Autodesk Inventor part; units mm, degrees
ref_plane "YZ Plane" through (0, 0, 0) normal (1, 0, 0) x (0, 1, 0)
ref_plane "XZ Plane" through (0, 0, 0) normal (0, 1, 0) x (-1, 0, 0)
ref_plane "XY Plane" through (0, 0, 0) normal (0, 0, 1) x (1, 0, 0)
sketch "Sketch1" plane through (0, 0, 0) normal (0, 0, 1) x (1, 0, 0)
  line L0 (-300, 620) -> (300, 620)
  line L1 (300, 620) -> (300, 0)
  line L2 (300, 0) -> (-300, 0)
  line L3 (-300, 0) -> (-300, 620)
  point P0 (0, 0)
  point P1 (0, 0)
  dimension "d0" = 600
  dimension "d1" = 620
extrude "Extrusion1" add sketch "Sketch1" along normal blind 400
sketch "Sketch2" plane through (0, 0, 400) normal (0, 0, 1) x (1, 0, 0)
  line L0 (-300, 0) -> (300, 0)
  line L1 (300, 0) -> (300, 620)
  line L2 (300, 620) -> (-300, 620)
  line L3 (-300, 620) -> (-300, 0)
  line L4 (-275, 595) -> (275, 595)
  line L5 (275, 595) -> (275, 421.6667)
  line L6 (275, 421.6667) -> (-275, 421.6667)
  line L7 (-275, 421.6667) -> (-275, 595)
  line L8 (275, 396.6667) -> (-275, 396.6667)
  line L9 (-275, 396.6667) -> (-275, 223.3333)
  line L10 (-275, 223.3333) -> (275, 223.3333)
  line L11 (275, 223.3333) -> (275, 396.6667)
  line L12 (-275, 198.3333) -> (275, 198.3333)
  line L13 (275, 198.3333) -> (275, 25)
  line L14 (275, 25) -> (-275, 25)
  line L15 (-275, 25) -> (-275, 198.3333)
  line L16 (-275, 421.6667) -> (-275, 396.6667) construction
  line L17 (-275, 223.3333) -> (-275, 198.3333) construction
  line L18 (-275, 595) -> (-300, 620) construction
  line L19 (275, 595) -> (300, 620) construction
  line L20 (-275, 25) -> (-300, 0) construction
  point P0 (0, 0)
  dimension "d4" = 25
  dimension "d5" = 25
extrude "Extrusion2" cut sketch "Sketch2" against normal blind 375 contours L4 L5 L6 L7 | L11 L10 L9 L8 | L12 L13 L14 L15
equation "\"d5\" = d4"
equation "\"d6\" = d2 - d4"
properties part number "Pensile"
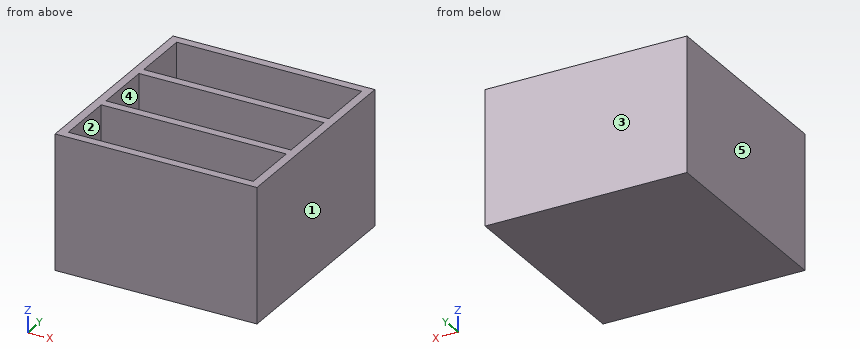
Geometry check sheet. Reference: the model listing, model coordinates, mm. Face numbers are marked on the shaded views. A direction names the side the tool comes from. Round coordinates to 2 decimals unless told otherwise and drop trailing zeros. Order: outer loops, then holes, each group sorted by start corner. A loop starts at its lowest first (then second) coordinate and runs counter-clockwise, first axis right, second up. Notation, with made-up numbers: M -19,-36 L 8,-36 A23 cw 8,-15 Z; hole C 35.25,13.25 d3. An arc over 180 degrees is marked long. Write item = value, one per line.
Q1. Set-up check for the marked faces 1 and 2: record each of +Z, -Z, +X, -X, +Y, -Y from which the full face is reachable in a straight line by a thin tool's end or side.
Answer block:
face_1 = +Z, -Z, +X, +Y, -Y
face_2 = +Z
Q2. Section check A-A (z = 374.5). Enter the section's corners in (x, y), plus the area to 3 significant figures.
Answer block:
outline = M -300,0 L 300,0 L 300,620 L -300,620 Z; hole M -275,25 L 275,25 L 275,198.33 L -275,198.33 Z; hole M -275,223.33 L 275,223.33 L 275,396.67 L -275,396.67 Z; hole M -275,421.67 L 275,421.67 L 275,595 L -275,595 Z
area = 86,000 mm^2
Q3. Scan lines: line 1 (Y direction, x = 206, z = 105); line 2 (X direction, y = 108.5, z = 122); line 3 (Z direction, x = -34, y = 349). Record each from-to range of solid material in increasing order.
Answer block:
line_1 = 0 to 25, 198.33 to 223.33, 396.67 to 421.67, 595 to 620
line_2 = -300 to -275, 275 to 300
line_3 = 0 to 25
Q4. Section check B-B (x = -15). Enter the section's corners in (y, z).
Answer block:
outline = M 0,0 L 620,0 L 620,400 L 595,400 L 595,25 L 421.67,25 L 421.67,400 L 396.67,400 L 396.67,25 L 223.33,25 L 223.33,400 L 198.33,400 L 198.33,25 L 25,25 L 25,400 L 0,400 Z
Q5. Section check C-C (y = 296). Enter the section's corners in (x, z).
Answer block:
outline = M -300,0 L 300,0 L 300,400 L 275,400 L 275,25 L -275,25 L -275,400 L -300,400 Z
Q6. Release check for a two-part mould opening along Y. For the marked faces 3, 4 and 5 record: released by +Y, released by -Y, zero draft, split by the parting line, or undercut.
Answer block:
face_3 = released by +Y
face_4 = undercut
face_5 = zero draft
